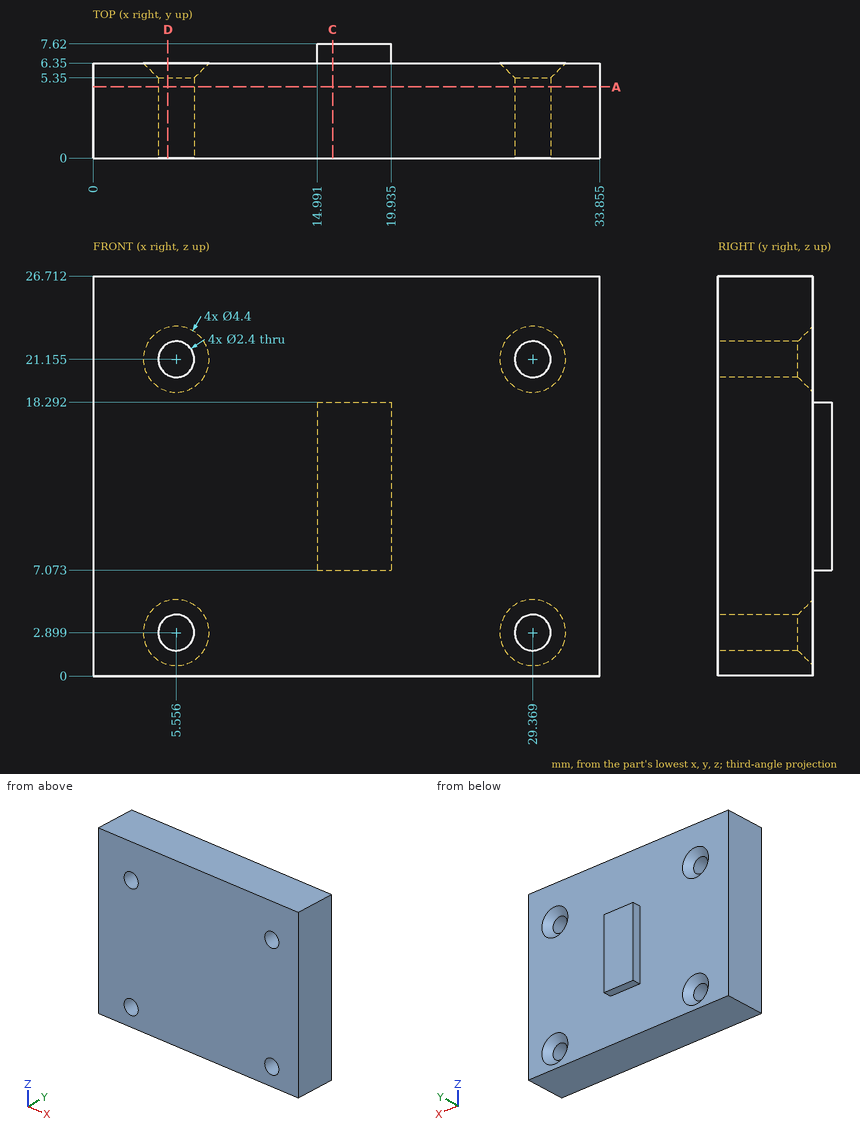
Input: dimensioned drawing with shaded views. Units: mm. Origin: part minimum x, y, z. Round coordinates to 2 decimals unless told otherwise and drop trailing zeros. Loops run counter-clockwise (first coordinate to the right, second up) from the corner with the lowest first, then second, coordinate; pieces in that order, holes last.
1) Pin query (flat end, axial travel): pin 1 (1 mm diameter, centred on x = 17, y = 7, fed in from -Z); pin 2 (0.6 mm diameter, centred on x = 17, y = 7, fed in from +Z); pin 3 (1.9 mm diameter, centred on x = 29.37, z = 21.16, fed in from -Y). Return the tip coordinate at first contact, or that it passes through.
Ans:
pin 1: stops at z = 7.07
pin 2: stops at z = 18.29
pin 3: passes through
2) Section query C-C on x = 16. Return the cut outline in (y, z).
Ans:
outline: (0, 0) - (6.35, 0) - (6.35, 7.07) - (7.62, 7.07) - (7.62, 18.29) - (6.35, 18.29) - (6.35, 26.71) - (0, 26.71) - close
3) Section query A-A on y = 4.75. Return the cut outline in (x, z) (1 decimal).
Ans:
outline: (0, 0) - (33.9, 0) - (33.9, 26.7) - (0, 26.7) - close; hole circle Ø2.4 at (5.6, 2.9); hole circle Ø2.4 at (5.6, 21.2); hole circle Ø2.4 at (29.4, 2.9); hole circle Ø2.4 at (29.4, 21.2)
4) Section query D-D on x = 5. Count the separate pieces of the cut face and the enclosed holes in it.
Ans:
separate pieces: 3
enclosed holes: 0
5) Material intervals for line 1 (Z direction, x = 6, y = 3.5) (1 decimal); line 2 (Z direction, x = 5, y = 0.5) (1 decimal); line 3 (X direction, y = 3.5, z = 3.5) (1 decimal), sorted ascending.
Ans:
line 1: z = 0 to 1.8, 4 to 20, 22.3 to 26.7
line 2: z = 0 to 1.8, 4 to 20.1, 22.2 to 26.7
line 3: x = 0 to 4.5, 6.6 to 28.3, 30.4 to 33.9
